from build123d import *

# Parameters (mm, degrees)
F0_W      = 304.8
F0_H      = 25.4
F1_DEPTH  = 19.05
F2_W      = 95.25
F2_H      = 25.4
F3_DEPTH  = 6.35
F4_W      = 95.25
F4_H      = 25.4
F5_DEPTH  = 6.35
F6_W      = 95.25
F6_H      = 25.4
F7_DEPTH  = 6.35
F8_W      = 95.25
F8_H      = 25.4
F9_DEPTH  = 6.35
F10_W     = 6.35
F10_H     = 76.2
F11_DEPTH = 25.4
F12_R     = 3.81
F13_DEPTH = 25.4
F14_W     = 25.961973
F14_H     = 114.3
F15_DEPTH = 6.35
F16_R     = 3.81
F17_DEPTH = 25.4
F18_R     = 3.81
F19_DEPTH = 25.4
F20_R     = 31.75
F21_DEPTH = 28.575
F22_R     = 25.4
F23_DEPTH = 22.225


with BuildPart() as f1:
    # F0 (on Right) → F1 (new body)
    with BuildSketch(Plane.YZ):
        with Locations((152.4, 12.7)):
            Rectangle(F0_W, F0_H)
    extrude(amount=F1_DEPTH)

    # F2 (on face) → F3 (cut)
    with BuildSketch(Plane.YZ.offset(19.05)):
        with Locations((47.625, 12.7)):
            Rectangle(F2_W, F2_H)
    extrude(amount=-F3_DEPTH, mode=Mode.SUBTRACT)

    # F4 (on face) → F5 (cut)
    with BuildSketch(Plane(origin=(0, 0, 0), x_dir=(0, -1, 0), z_dir=(-1, 0, 0))):
        with Locations((-47.625, 12.7)):
            Rectangle(F4_W, F4_H)
    extrude(amount=-F5_DEPTH, mode=Mode.SUBTRACT)

    # F6 (on face) → F7 (cut)
    with BuildSketch(Plane.YZ.offset(19.05)):
        with Locations((257.175, 12.7)):
            Rectangle(F6_W, F6_H)
    extrude(amount=-F7_DEPTH, mode=Mode.SUBTRACT)

    # F8 (on face) → F9 (cut)
    with BuildSketch(Plane(origin=(0, 0, 0), x_dir=(0, -1, 0), z_dir=(-1, 0, 0))):
        with Locations((-257.175, 12.7)):
            Rectangle(F8_W, F8_H)
    extrude(amount=-F9_DEPTH, mode=Mode.SUBTRACT)

    # F10 (on face) → F11 (cut)
    with BuildSketch(Plane.XY.offset(25.4)):
        with Locations((9.525, 152.4)):
            Rectangle(F10_W, F10_H)
    extrude(amount=-F11_DEPTH, mode=Mode.SUBTRACT)

    # F12 (on face) → F13 (cut)
    with BuildSketch(Plane.YZ.offset(19.05)):
        with Locations((152.4, 12.7)):
            Circle(F12_R)
    extrude(amount=-F13_DEPTH, mode=Mode.SUBTRACT)

    # F14 (on face) → F15 (join)
    with BuildSketch(Plane.XY.offset(25.4)):
        with Locations((9.805986, 314.325)):
            Rectangle(F14_W, F14_H)
    extrude(amount=F15_DEPTH)

    # F16 (on face) → F17 (cut)
    with BuildSketch(Plane.XY.offset(31.75)):
        with Locations((10.086973, 313.690683)):
            Circle(F16_R)
    extrude(amount=-F17_DEPTH, mode=Mode.SUBTRACT)

    # F18 (on face) → F19 (cut)
    with BuildSketch(Plane.YZ.offset(12.7)):
        with Locations((53.975, 12.7)):
            Circle(F18_R)
    extrude(amount=-F19_DEPTH, mode=Mode.SUBTRACT)

    # F20 (on face) → F21 (join)
    with BuildSketch(Plane.XY.offset(31.75)):
        with Locations((9.805986, 361.007124)):
            Circle(F20_R)
    extrude(amount=F21_DEPTH)

    # F22 (on face) → F23 (cut)
    with BuildSketch(Plane.XY.offset(60.325)):
        with Locations((9.805986, 361.007124)):
            Circle(F22_R)
    extrude(amount=-F23_DEPTH, mode=Mode.SUBTRACT)


solid = f1.part
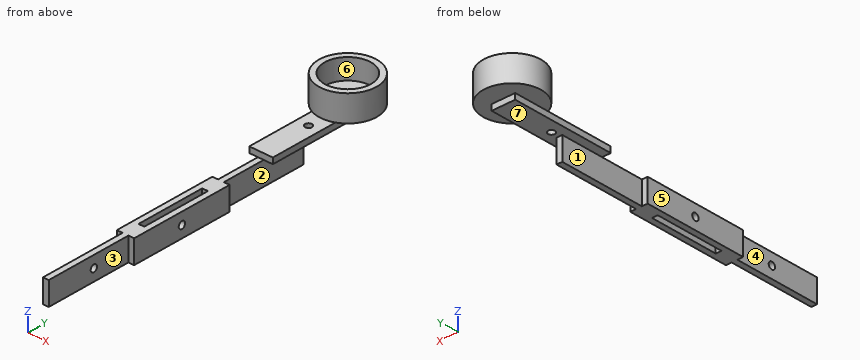
Read the model definition and answer for the solid it produces. Units are mm, in the model's axes. Face numbers are marked on the shaded views. A direction names the side the tool comes from. Coordinates: 2 decimals unless noted, no trailing zeros. Loops run counter-clockwise (first coordinate to the right, second up) from the corner with the lowest first, then second, coordinate; pieces in that order, holes last. Notation, with made-up numbers: (-27.5, 13) - (-13.5, 13) arc R29 ccw to (-13.5, 52) - close; hole circle Ø10 at (-7.5, -11.75). An arc over 180 degrees is marked (long way). Answer in a Markdown table with one row per item.
Q1. For the marked faces 1, 2, 3 and 4, determine the directions among +Z, -Z, +X, -X, +Y, -Y from which every point of the face is accessible in a straight line to the end or side of a thin tool.
Here are the results:
| item | result |
|---|---|
| face 1 | -Z, -X, +Y |
| face 2 | -Z, +X, +Y |
| face 3 | +Z, -Z, +X, -Y |
| face 4 | +Z, -Z, -X, -Y |
Q2. Find section D-D on x = -9.5. Write down the section's boundary in (y, z) (3 decimals), plus the area to 3 significant figures.
Here are the results:
| item | result |
|---|---|
| outline | (335.801, 31.75) - (386.213, 31.75) - (386.213, 60.325) - (377.513, 60.325) - (377.513, 38.1) - (344.501, 38.1) - (344.501, 60.325) - (335.801, 60.325) - close |
| area | 707 mm^2 |
Q3. Find section A-A on y = 166.5. Write down the section's boundary in (x, z), plus the area to 3 significant figures.
Here are the results:
| item | result |
|---|---|
| outline | (0, 0) - (6.35, 0) - (6.35, 25.4) - (0, 25.4) - close; (12.7, 0) - (19.05, 0) - (19.05, 25.4) - (12.7, 25.4) - close |
| area | 323 mm^2 |
Q4. Given P1, Ø5, axis at x = 17, z = 46.5, coming from the +Y side; P2, Ø12.5, axis at y = 260, z = 18.5, coming from the +X side; P3, Ø1.9, axis at x = 4, z = 9.5, coming from the +Y side, each flat-ended and moving along its own axis, determine where each tip first touches the part or whether it passes through.
Here are the results:
| item | result |
|---|---|
| P1 | stops at y = 392.41 |
| P2 | stops at x = 12.7 |
| P3 | stops at y = 209.55 |
Q5. The mould has two halves that part along X. Classify the marked faces 5, 6 and 7: pulls with the +X half, pulls with the -X half, needs draft (parallel to the pull), parting line crosses it, or undercut.
Here are the results:
| item | result |
|---|---|
| face 5 | pulls with the -X half |
| face 6 | undercut |
| face 7 | needs draft |
Q6. Find section C-C on y = 273.5. Write down the section's boundary in (x, z) (3 decimals).
Here are the results:
| item | result |
|---|---|
| outline | (-3.175, 25.4) - (6.35, 25.4) - (6.35, 0) - (12.7, 0) - (12.7, 25.4) - (22.787, 25.4) - (22.787, 31.75) - (-3.175, 31.75) - close |
Q7. Straight lines are drawn through the part: line 1 along Z through (x, y) = (2, 152); line 2 along Y through (x, z) = (9, 12); line 3 along Y through (x, z) = (14, 12). For each, find the intervals that lie inside material, in ascending order. Write a range as [from, to].
Here are the results:
| item | result |
|---|---|
| line 1 | z = [0, 8.91], [16.49, 25.4] |
| line 2 | y = [0, 50.23], [57.72, 114.3], [190.5, 304.8] |
| line 3 | y = [95.25, 148.65], [156.15, 209.55] |
Q8. Find section B-B on z = 12.7. Write down the section's boundary in (x, y) (3 decimals).
Here are the results:
| item | result |
|---|---|
| outline | (0, 95.25) - (6.35, 95.25) - (6.35, 57.785) - (12.7, 57.785) - (12.7, 95.25) - (19.05, 95.25) - (19.05, 148.59) - (12.7, 148.59) - (12.7, 114.3) - (6.35, 114.3) - (6.35, 148.59) - (0, 148.59) - close; (0, 156.21) - (6.35, 156.21) - (6.35, 190.5) - (12.7, 190.5) - (12.7, 156.21) - (19.05, 156.21) - (19.05, 209.55) - (12.7, 209.55) - (12.7, 304.8) - (6.35, 304.8) - (6.35, 209.55) - (0, 209.55) - close; (6.35, 0) - (12.7, 0) - (12.7, 50.165) - (6.35, 50.165) - close |
